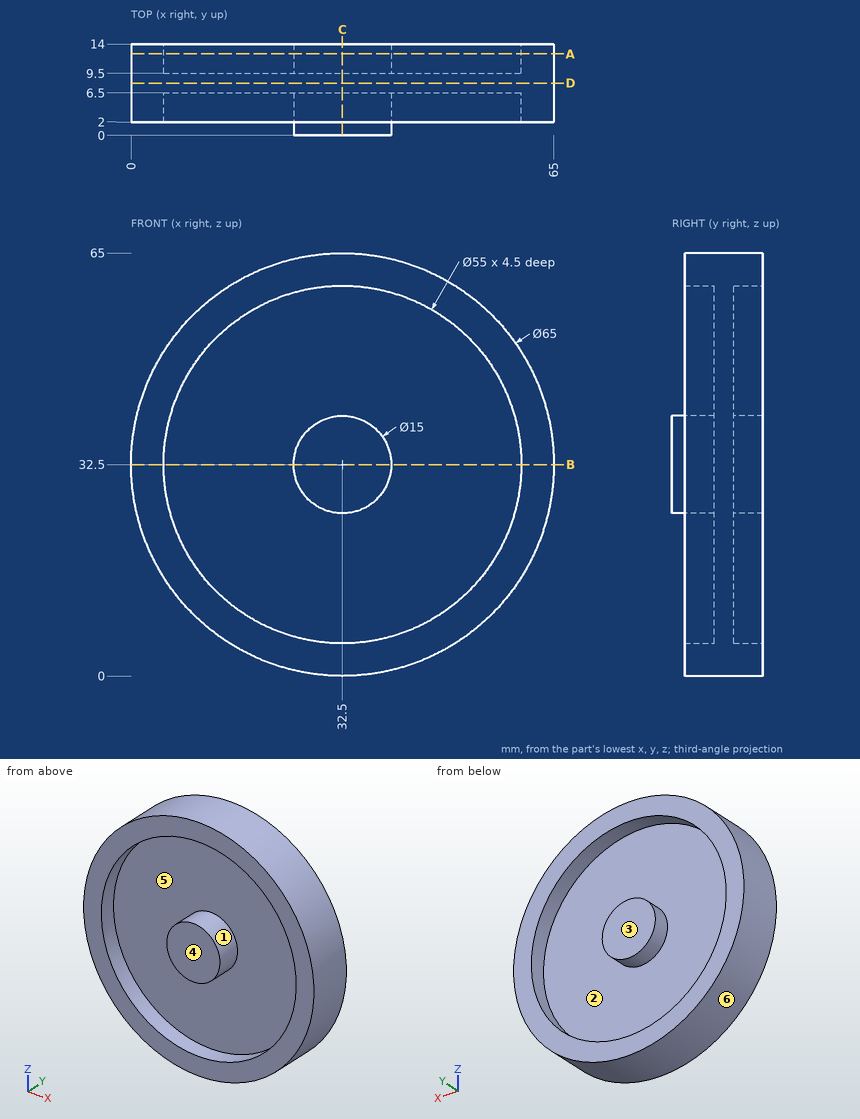
For this review, use the dimensioned drawing (mm, ordinates from the lowest corner) and the shaded views. A direction names the side the tool comes from. Coordinates: 2 decimals unless noted, no trailing zeros. Order: outer loops, then holes, each group sorted by start corner. A loop starts at its lowest first (then second) coordinate and runs counter-clockwise, first axis right, second up. Notation, with made-up numbers: (5, 25) - (18, 25) arc R35 cw to (18, 60) - close; hole circle Ø3 at (-31, -17). An arc over 180 degrees is marked (long way). Answer as a JSON object with one key per item and string values. Group by question number.
1. We need section D-D on y = 8. State the section outline as (x, z) points, then the cut area to 3 significant figures.
2. We need section C-C on x = 32.5. State the section outline as (y, z) points, then the cut area to 3 significant figures.
3. Clearance check with flat-ended pins moving along their axes: P1, Ø6, axis at x = 38.5, z = 11, coming from the -Y side; P2, Ø3, axis at x = 56, z = 18.5, coming from the -Y side; P3, Ø8, axis at x = 21, z = 25, coming from the +Y side. State where each tip first meets the part, or that it passes through.
4. We need section B-B on z = 32.5. State the section outline as (x, y) points.
5. We need section A-A on y = 12.5. State the section outline as (x, z) points.
6. The part is to be moulded in two halves that separate along Z. For the marked faces 4, 5 and 6, say which applies: pulls with the +Z half, pulls with the -Z half, needs draft (parallel to the pull), parting line crosses it, or undercut.
7. For the marked faces 1, 2 and 3, list the 3-axis set-ups (+Z, -Z, +X, -X, +Y, -Y) from which the entire face can be reached by the end or side of a thin tool; tool diameter is ignored.
8. For probe 1 along X at (y, z) = (5, 32.5); probe 2 along Z at (x, y) = (35, 11); probe 3 along Z at (x, y) = (31, 12.5), list the stretches that pass through material, from the lowest coordinate up.
Final values:
{
 "1": {"outline": "circle Ø65 at (32.5, 32.5)", "area": "3,320 mm²"},
 "2": {"outline": "(0, 25) - (6.5, 25) - (6.5, 5) - (2, 5) - (2, 0) - (14, 0) - (14, 5) - (9.5, 5) - (9.5, 25) - (14, 25) - (14, 40) - (9.5, 40) - (9.5, 60) - (14, 60) - (14, 65) - (2, 65) - (2, 60) - (6.5, 60) - (6.5, 40) - (0, 40) - close", "area": "450 mm²"},
 "3": {"P1": "y = 6.5", "P2": "y = 2", "P3": "y = 9.5"},
 "4": {"outline": "(0, 2) - (5, 2) - (5, 6.5) - (25, 6.5) - (25, 0) - (40, 0) - (40, 6.5) - (60, 6.5) - (60, 2) - (65, 2) - (65, 14) - (60, 14) - (60, 9.5) - (40, 9.5) - (40, 14) - (25, 14) - (25, 9.5) - (5, 9.5) - (5, 14) - (0, 14) - close"},
 "5": {"outline": "circle Ø65 at (32.5, 32.5); circle Ø15 at (32.5, 32.5); hole circle Ø55 at (32.5, 32.5)"},
 "6": {"face 4": "needs draft", "face 5": "undercut", "face 6": "parting line crosses it"},
 "7": {"face 1": "-Y", "face 2": "+Y", "face 3": "+Z, -Z, +X, -X, +Y"},
 "8": {"probe 1": "0 to 5, 25 to 40, 60 to 65", "probe 2": "0.1 to 5.11, 25.43 to 39.57, 59.89 to 64.9", "probe 3": "0.03 to 5.04, 25.15 to 39.85, 59.96 to 64.97"}
}
